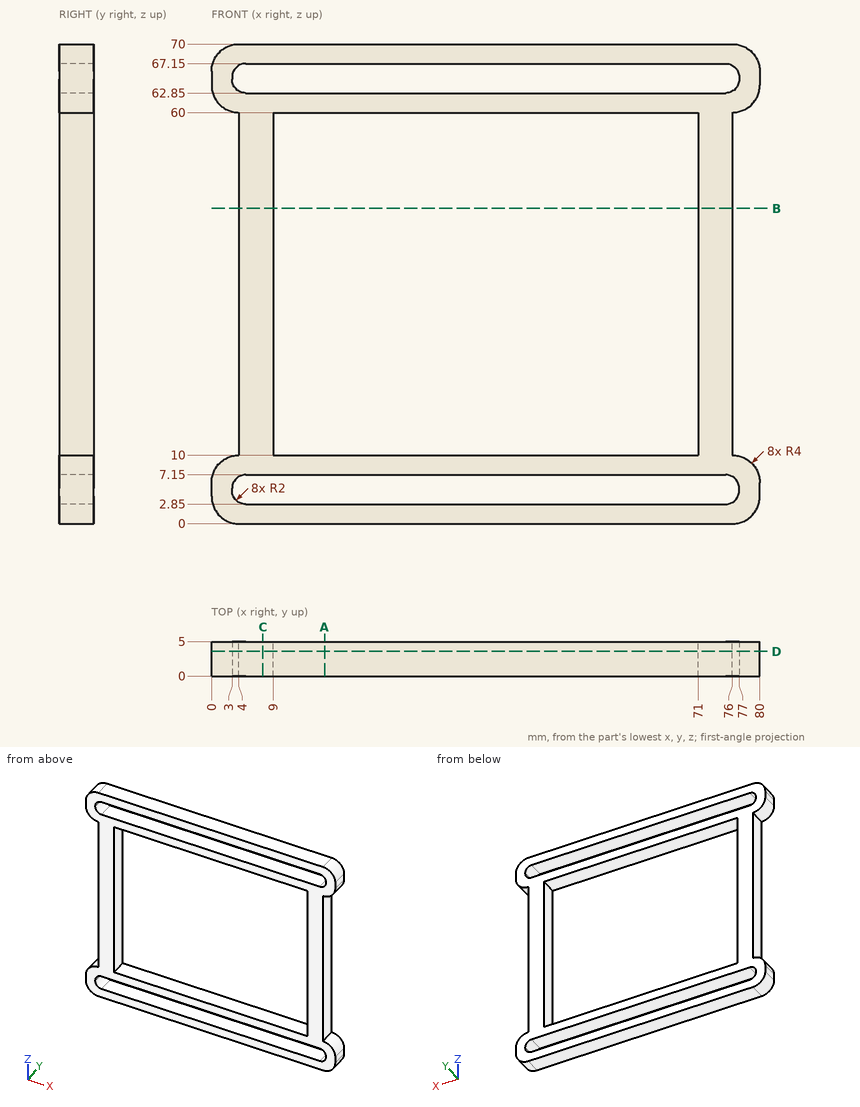
Answer from the drawing. Dimensions are ordinates in mm from the lowest x, y and z of the part. Give positions to 0.01 mm unless a question says otherwise; leave off trailing zeros. Loops run counter-clockwise (first coordinate to the right, second up) from the corner with the lowest first, then second, coordinate; pieces in that order, holes last. Notation, with made-up numbers: (-24.75, 47) -> (20.25, 47) arc R24 ccw to (20.25, 85) -> close; hole circle Ø5 at (4.25, -12.75). An arc over 180 degrees is marked (long way). Answer as CSV lines item,"result".
Item 1: Find section A-A on x = 16.5. Give the vertices of the cut face in (y, z).
Returned:
outline,"(0, 0) -> (5, 0) -> (5, 2.85) -> (0, 2.85) -> close; (0, 7.15) -> (5, 7.15) -> (5, 10) -> (0, 10) -> close; (0, 60) -> (5, 60) -> (5, 62.85) -> (0, 62.85) -> close; (0, 67.15) -> (5, 67.15) -> (5, 70) -> (0, 70) -> close"
Item 2: Find section B-B on z = 46. Give the vertices of the cut face in (x, y).
Returned:
outline,"(4, 0) -> (9, 0) -> (9, 5) -> (4, 5) -> close; (71, 0) -> (76, 0) -> (76, 5) -> (71, 5) -> close"
Item 3: Each of these flat-tipped pins is pushed along its axis until it touches: pin 1 (2.5 mm diameter, centred on y = 3.5, z = 43.5, fed in from +X); pin 2 (1.5 mm diameter, centred on y = 2.5, z = 40, fed in from -X); pin 3 (6 mm diameter, centred on x = 35.5, z = 54.5, fed in from -Y). Where does it stop, or does it pass through?
Returned:
pin 1,"stops at x = 76"
pin 2,"stops at x = 4"
pin 3,"passes through"
Item 4: Consider line 1 (Z direction, x = 29.5, y = 1.85); line 2 (Z direction, x = 73, y = 3.65); line 3 (X direction, y = 3, z = 14). Determine where each line is inside the solid, lowest interval first. Write a range as [from, to].
Returned:
line 1,"z = [0, 2.85], [7.15, 10], [60, 62.85], [67.15, 70]"
line 2,"z = [0, 2.85], [7.15, 62.85], [67.15, 70]"
line 3,"x = [4, 9], [71, 76]"
Item 5: Find section C-C on x = 7.5. Give the vertices of the cut face in (y, z).
Returned:
outline,"(0, 0) -> (5, 0) -> (5, 2.85) -> (0, 2.85) -> close; (0, 7.15) -> (5, 7.15) -> (5, 62.85) -> (0, 62.85) -> close; (0, 67.15) -> (5, 67.15) -> (5, 70) -> (0, 70) -> close"
Item 6: Find section D-D on y = 3.6. State how many separate pieces and enclosed holes the cut face has, plus the area to 3 significant figures.
Returned:
separate pieces,"1"
enclosed holes,"3"
area,"1,440 mm²"
